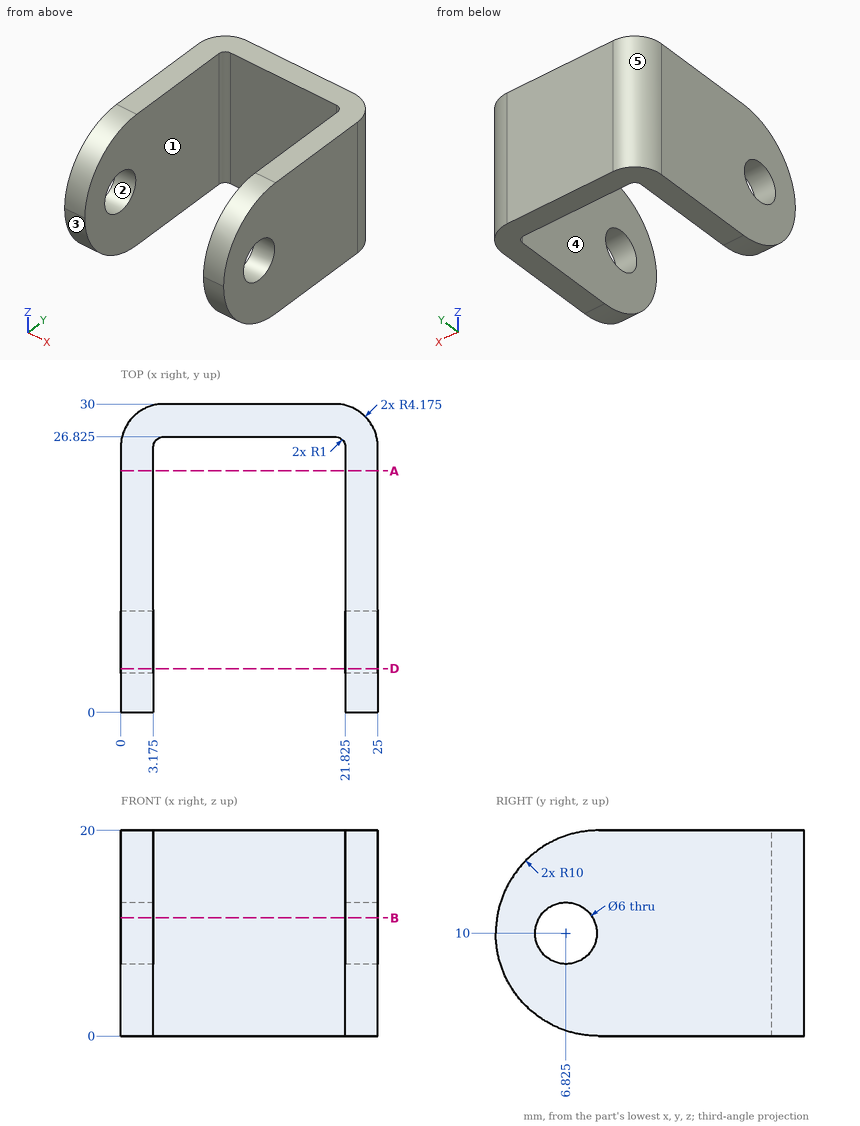
Study the drawing (mm; zero at the part's minimum x, y, z) and answer. A direction names the side the tool comes from. Give positions to 0.01 mm unless a question says otherwise; leave off trailing zeros. Write each loop counter-clockwise with the first axis right and the second up, starting at its lowest first coordinate (ties: lowest second). Pieces come first, ordered by that corner, then holes. Notation, with made-up numbers: (14.5, -16) -> (71.5, -16) arc R32 cw to (71.5, 15) -> close; hole circle Ø1 at (-11.75, -16). An arc over 180 degrees is marked (long way). Answer as a JSON object with one key per item and string values. Group by question number.
1) Consider L1, parallel to X at y = 20.5, z = 14.5 (3 decimals); L2, parallel to Y at x = 2.1, z = 10 (1 decimal); L3, parallel to Z at x = 24, y = 8. Determine where each line is inside the solid, lowest interval first. Write a range as from..to.
2) Find section D-D (y = 4.25). Write down the section's boundary in (x, z) (1 decimal).
3) Each of these flat-tipped pins is pushed along its axis until it touches: P1, Ø8, axis at x = 4.5, z = 17, coming from the -Y side; P2, Ø8.5, axis at x = 8.5, z = 12.5, coming from the -Y side (3 decimals). Where does it stop, or does it pass through?
4) Find section B-B (z = 11.5). Write down the section's boundary in (x, y) (3 decimals).
5) The mould has two halves that part along X. Classify the marked faces 3, 4 and 5: +X half, -X half, draft (parallel to the pull), parting line (faces both ways), or undercut.
6) Find section A-A (y = 23.5). Write down the section's boundary in (x, z) (3 decimals), and give its area (3 significant figures).
7) A tool of negligible diameter and unlimited length cuts with its end or side. For the marked faces 1 and 2, from which of +Z, -Z, +X, -X, +Y, -Y can it reach the whole face along a straight path? Write none if from no direction.
Values follow:
{
 "1": {"L1": "x = 0..3.175, 21.825..25", "L2": "y = 0..3.8, 9.8..29.4", "L3": "z = 0.2..7.24, 12.76..19.8"},
 "2": {"outline": "(0, 1.8) -> (3.2, 1.8) -> (3.2, 8.5) -> (0, 8.5) -> close; (0, 11.5) -> (3.2, 11.5) -> (3.2, 18.2) -> (0, 18.2) -> close; (21.8, 1.8) -> (25, 1.8) -> (25, 8.5) -> (21.8, 8.5) -> close; (21.8, 11.5) -> (25, 11.5) -> (25, 18.2) -> (21.8, 18.2) -> close"},
 "3": {"P1": "stops at y = 0.53", "P2": "stops at y = 26.825"},
 "4": {"outline": "(0, 0.113) -> (3.175, 0.113) -> (3.175, 4.227) -> (0, 4.227) -> close; (0, 9.423) -> (3.175, 9.423) -> (3.175, 25.825) arc R1 cw to (4.175, 26.825) -> (20.825, 26.825) arc R1 cw to (21.825, 25.825) -> (21.825, 9.423) -> (25, 9.423) -> (25, 25.825) arc R4.175 ccw to (20.825, 30) -> (4.175, 30) arc R4.175 ccw to (0, 25.825) -> close; (21.825, 0.113) -> (25, 0.113) -> (25, 4.227) -> (21.825, 4.227) -> close"},
 "5": {"face 3": "draft", "face 4": "undercut", "face 5": "-X half"},
 "6": {"outline": "(0, 0) -> (3.175, 0) -> (3.175, 20) -> (0, 20) -> close; (21.825, 0) -> (25, 0) -> (25, 20) -> (21.825, 20) -> close", "area": "127 mm2"},
 "7": {"face 1": "+Z, -Z, -Y", "face 2": "+X, -X"}
}
